Could you check a few things on this model? Use its own coordinates, in mm. A direction names the side the tool comes from. Round coordinates to 2 decimals unless told otherwise and drop trailing zeros. Loops run counter-clockwise (first coordinate to the right, second up) from the corner with the lowest first, then second, coordinate; pieces in that order, holes last. Notation, with made-up numbers: M -5.5,85 L 20.5,85 A20 ccw 20.5,103 Z; hole C 51.25,-19 d4. An arc over 180 degrees is marked long. Answer in a Markdown table with one row per item.
```python
from build123d import *

# Parameters (mm, degrees)
BASE_FLANGE1_DEPTH           = 1
SKETCH6_R                    = 6.5
CUT_EXTRUDE1_DEPTH           = 10
EDGE_FLANGE1_STRIP_W         = 10
EDGE_FLANGE1_STRIP_H         = 1
EDGE_FLANGE1_STRIP_CUT_DEPTH = 32
EDGE_FLANGE1_DEPTH           = 32
EDGE_FLANGE2_STRIP_W         = 10
EDGE_FLANGE2_STRIP_H         = 1
EDGE_FLANGE2_STRIP_CUT_DEPTH = 32
EDGE_FLANGE2_DEPTH           = 32
EDGE_FLANGE2_FLAT_DEPTH      = 1
EDGE_FLANGE3_STRIP_W         = 10
EDGE_FLANGE3_STRIP_H         = 1
EDGE_FLANGE3_STRIP_CUT_DEPTH = 8
EDGE_FLANGE3_DEPTH           = 8
EDGE_FLANGE4_STRIP_W         = 10
EDGE_FLANGE4_STRIP_H         = 1
EDGE_FLANGE4_STRIP_CUT_DEPTH = 25
EDGE_FLANGE4_DEPTH           = 25
EDGE_FLANGE4_FLAT_DEPTH      = 1
EDGE_FLANGE5_STRIP_W         = 10
EDGE_FLANGE5_STRIP_H         = 1
EDGE_FLANGE5_STRIP_CUT_DEPTH = 19
EDGE_FLANGE5_DEPTH           = 19
EDGE_FLANGE5_PROFILE_W       = 19
EDGE_FLANGE5_PROFILE_H       = 26
EDGE_FLANGE5_PROFILE_R       = 4
EDGE_FLANGE5_FLAT_DEPTH      = 1


# Sheet-metal steps are written as plain solids
with BuildPart() as part:
    # Sketch1 → Base-Flange1 (new body)
    with BuildSketch(Plane.XY):
        with BuildLine():
            Line((-47.5, 0), (47.5, 0))
            Line((47.5, 0), (47.5, -32))
            Line((47.5, -32), (31.5, -32))
            ThreePointArc((31.5, -32), (28.671572875, -33.171572875), (27.5, -36))
            Line((27.5, -36), (27.5, -44))
            Line((27.5, -44), (2.5, -44))
            Line((2.5, -44), (2.5, -30))
            ThreePointArc((2.5, -30), (1.328427125, -27.171572875), (-1.5, -26))
            Line((-1.5, -26), (-13.5, -26))
            ThreePointArc((-13.5, -26), (-16.328427125, -27.171572875), (-17.5, -30))
            Line((-17.5, -30), (-17.5, -44))
            Line((-17.5, -44), (-25.5, -44))
            Line((-25.5, -44), (-25.5, -36))
            ThreePointArc((-25.5, -36), (-26.671572875, -33.171572875), (-29.5, -32))
            Line((-29.5, -32), (-47.5, -32))
            Line((-47.5, -32), (-47.5, 0))
        make_face()
    extrude(amount=-BASE_FLANGE1_DEPTH)

    # Sketch6 → Cut-Extrude1 (cut)
    with BuildSketch(Plane.XY):
        with Locations((21, -22)):
            Circle(SKETCH6_R)
    extrude(amount=-CUT_EXTRUDE1_DEPTH, mode=Mode.SUBTRACT)

    # Edge-Flange1 strip (across the edge) → Edge-Flange1 strip cut (cut)
    with BuildSketch(Plane(origin=(47.5, 0, -1), x_dir=(-1, 0, 0), z_dir=(0, -1, 0))):
        with Locations((-1, -0.5)):
            Rectangle(EDGE_FLANGE1_STRIP_W, EDGE_FLANGE1_STRIP_H)
    edge_flange1_strip_cut = extrude(amount=EDGE_FLANGE1_STRIP_CUT_DEPTH, mode=Mode.SUBTRACT)

    # Edge-Flange1 section (across the edge) → Edge-Flange1 (add)
    with BuildSketch(Plane(origin=(47.5, 0, -1), x_dir=(-1, 0, 0), z_dir=(0, -1, 0))):
        with BuildLine():
            Line((0, 3), (0, 40))
            Line((0, 40), (1, 40))
            Line((1, 40), (1, 3))
            ThreePointArc((1, 3), (1.878679656, 0.878679656), (4, 0))
            Line((4, 0), (4, -1))
            ThreePointArc((4, -1), (1.171572875, 0.171572875), (0, 3))
        make_face()
    edge_flange1 = extrude(amount=EDGE_FLANGE1_DEPTH)

    # Edge-Flange2 strip (across the edge) → Edge-Flange2 strip cut (cut)
    with BuildSketch(Plane(origin=(47.5, -32, -41), x_dir=(0, 0, 1), z_dir=(0, 1, 0))):
        with Locations((-1, -0.5)):
            Rectangle(EDGE_FLANGE2_STRIP_W, EDGE_FLANGE2_STRIP_H)
    edge_flange2_strip_cut = extrude(amount=EDGE_FLANGE2_STRIP_CUT_DEPTH, mode=Mode.SUBTRACT)

    # Edge-Flange2 bend section (across the edge) → Edge-Flange2 (add)
    with BuildSketch(Plane(origin=(47.5, -32, -41), x_dir=(0, 0, 1), z_dir=(0, 1, 0))):
        with BuildLine():
            Line((0, 3), (1, 3))
            ThreePointArc((1, 3), (1.878679656, 0.878679656), (4, 0))
            Line((4, 0), (4, -1))
            ThreePointArc((4, -1), (1.171572875, 0.171572875), (0, 3))
        make_face()
    edge_flange2 = extrude(amount=EDGE_FLANGE2_DEPTH)

    # Edge-Flange2 profile (on flange) → Edge-Flange2 flat (add)
    with BuildSketch(Plane(origin=(47.5, 0, -41), x_dir=(0, 1, 0), z_dir=(0, 0, -1))):
        with BuildLine():
            Line((-32, 3), (0, 3))
            Line((0, 3), (0, 14))
            ThreePointArc((0, 14), (-2.050252532, 18.949747468), (-7, 21))
            Line((-7, 21), (-25, 21))
            ThreePointArc((-25, 21), (-29.949747468, 18.949747468), (-32, 14))
            Line((-32, 14), (-32, 3))
        make_face()
    edge_flange2_flat = extrude(amount=-EDGE_FLANGE2_FLAT_DEPTH)

    # Mirror1: Edge-Flange1 strip cut, Edge-Flange1, Edge-Flange2 strip cut, Edge-Flange2, Edge-Flange2 flat across plane
    add(edge_flange1_strip_cut.mirror(Plane(origin=(0, 0, 0), x_dir=(0, 0, 1), z_dir=(1, 0, 0))), mode=Mode.SUBTRACT)
    add(edge_flange1.mirror(Plane(origin=(0, 0, 0), x_dir=(0, 0, 1), z_dir=(1, 0, 0))))
    add(edge_flange2_strip_cut.mirror(Plane(origin=(0, 0, 0), x_dir=(0, 0, 1), z_dir=(1, 0, 0))), mode=Mode.SUBTRACT)
    add(edge_flange2.mirror(Plane(origin=(0, 0, 0), x_dir=(0, 0, 1), z_dir=(1, 0, 0))))
    add(edge_flange2_flat.mirror(Plane(origin=(0, 0, 0), x_dir=(0, 0, 1), z_dir=(1, 0, 0))))

    # Edge-Flange3 strip (across the edge) → Edge-Flange3 strip cut (cut)
    with BuildSketch(Plane(origin=(-17.5, -44, -1), x_dir=(0, 1, 0), z_dir=(-1, 0, 0))):
        with Locations((-1, -0.5)):
            Rectangle(EDGE_FLANGE3_STRIP_W, EDGE_FLANGE3_STRIP_H)
    extrude(amount=EDGE_FLANGE3_STRIP_CUT_DEPTH, mode=Mode.SUBTRACT)

    # Edge-Flange3 section (across the edge) → Edge-Flange3 (add)
    with BuildSketch(Plane(origin=(-17.5, -44, -1), x_dir=(0, 1, 0), z_dir=(-1, 0, 0))):
        with BuildLine():
            Line((0, 3), (0, 18))
            Line((0, 18), (1, 18))
            Line((1, 18), (1, 3))
            ThreePointArc((1, 3), (1.878679656, 0.878679656), (4, 0))
            Line((4, 0), (4, -1))
            ThreePointArc((4, -1), (1.171572875, 0.171572875), (0, 3))
        make_face()
    extrude(amount=EDGE_FLANGE3_DEPTH)

    # Edge-Flange4 strip (across the edge) → Edge-Flange4 strip cut (cut)
    with BuildSketch(Plane(origin=(27.5, -44, -1), x_dir=(0, 1, 0), z_dir=(-1, 0, 0))):
        with Locations((-1, -0.5)):
            Rectangle(EDGE_FLANGE4_STRIP_W, EDGE_FLANGE4_STRIP_H)
    extrude(amount=EDGE_FLANGE4_STRIP_CUT_DEPTH, mode=Mode.SUBTRACT)

    # Edge-Flange4 bend section (across the edge) → Edge-Flange4 (add)
    with BuildSketch(Plane(origin=(27.5, -44, -1), x_dir=(0, 1, 0), z_dir=(-1, 0, 0))):
        with BuildLine():
            Line((0, 3), (1, 3))
            ThreePointArc((1, 3), (1.878679656, 0.878679656), (4, 0))
            Line((4, 0), (4, -1))
            ThreePointArc((4, -1), (1.171572875, 0.171572875), (0, 3))
        make_face()
    extrude(amount=EDGE_FLANGE4_DEPTH)

    # Edge-Flange4 profile (on flange) → Edge-Flange4 flat (add)
    with BuildSketch(Plane(origin=(0, -44, -1), x_dir=(-1, 0, 0), z_dir=(0, -1, 0))):
        Polygon((-27.5, 3), (-2.5, 3), (-2.5, 8), (10.5, 8), (10.5, 14.535898385), (4.5, 18), (-2.5, 18), (-8.5, 18), (-8.5, 50), (-27.5, 50), align=None)
    extrude(amount=-EDGE_FLANGE4_FLAT_DEPTH)

    # Edge-Flange5 strip (across the edge) → Edge-Flange5 strip cut (cut)
    with BuildSketch(Plane(origin=(27.5, -43, -51), x_dir=(0, 0, 1), z_dir=(-1, 0, 0))):
        with Locations((-1, -0.5)):
            Rectangle(EDGE_FLANGE5_STRIP_W, EDGE_FLANGE5_STRIP_H)
    extrude(amount=EDGE_FLANGE5_STRIP_CUT_DEPTH, mode=Mode.SUBTRACT)

    # Edge-Flange5 bend section (across the edge) → Edge-Flange5 (add)
    with BuildSketch(Plane(origin=(27.5, -43, -51), x_dir=(0, 0, 1), z_dir=(-1, 0, 0))):
        with BuildLine():
            Line((0, 3), (1, 3))
            ThreePointArc((1, 3), (1.878679656, 0.878679656), (4, 0))
            Line((4, 0), (4, -1))
            ThreePointArc((4, -1), (1.171572875, 0.171572875), (0, 3))
        make_face()
    extrude(amount=EDGE_FLANGE5_DEPTH)

    # Edge-Flange5 profile (on flange) → Edge-Flange5 flat (add)
    with BuildSketch(Plane(origin=(0, -43, -51), x_dir=(-1, 0, 0), z_dir=(0, 0, -1))):
        with Locations((-18, 16)):
            Rectangle(EDGE_FLANGE5_PROFILE_W, EDGE_FLANGE5_PROFILE_H)
        with Locations((-18, 21)):
            Circle(EDGE_FLANGE5_PROFILE_R, mode=Mode.SUBTRACT)
    extrude(amount=-EDGE_FLANGE5_FLAT_DEPTH)


solid = part.part
```
1) I want a section at B-B, the plane x = 18. Please give me the cut outline in (y, z), plus the area to 3 significant figures.
Computed:
| item | result |
|---|---|
| outline | M -44,-47 A4 ccw -40,-51 L -26,-51 L -26,-50 L -40,-50 A3 cw -43,-47 L -43,-4 A3 cw -40,-1 L -27.77,-1 L -27.77,0 L -40,0 A4 ccw -44,-4 Z; M -18,-51 L -14,-51 L -14,-50 L -18,-50 Z; M -16.23,-1 L 0,-1 L 0,0 L -16.23,0 Z |
| area | 100 mm² |
2) I need wall thicknesses on line 1 (X direction, y = -19.5, z = -17); line 2 (Z direction, x = 63.5, y = -22.5); line 3 (Z direction, x = -4, y = -5). Which ranges of each line are inside material? Lowest first, please.
Computed:
| item | result |
|---|---|
| line 1 | x = -47.5 to -46.5, 46.5 to 47.5 |
| line 2 | z = -41 to -40 |
| line 3 | z = -1 to 0 |
3) If we mould it in two halves opening along Y, with no side actions, what happens to faces 4 (the face through (-66.5, -29.9, -40.5)), 5 (the face through (18.521, -18.034, -50.507)), 6 (the face through (18, -27, -51))? For each: released by +Y, released by -Y, zero draft, split by the parting line, or undercut.
Computed:
| item | result |
|---|---|
| face 4 | released by -Y |
| face 5 | undercut |
| face 6 | zero draft |
4) I want a section at D-D, the plane y = -4. Please give me the cut outline in (x, z).
Computed:
| item | result |
|---|---|
| outline | M -67.82,-41 L -50.5,-41 A4 ccw -46.5,-37 L -46.5,-4 A3 cw -43.5,-1 L 43.5,-1 A3 cw 46.5,-4 L 46.5,-37 A4 ccw 50.5,-41 L 67.82,-41 L 67.82,-40 L 50.5,-40 A3 cw 47.5,-37 L 47.5,-4 A4 ccw 43.5,0 L -43.5,0 A4 ccw -47.5,-4 L -47.5,-37 A3 cw -50.5,-40 L -67.82,-40 Z |
5) Will these pins go through, and if not, where does the flat tip stop? P1, Ø20, axis at x = 55.5, y = -17, coming from the +Z side; P2, Ø2, axis at y = -31, z = -14, coming from the +X side; P3, Ø12, axis at x = -14.5, y = -21, coming from the -Z side; P4, Ø8, axis at x = 47, z = -14, coming from the +Y side.
Computed:
| item | result |
|---|---|
| P1 | stops at z = -0.54 |
| P2 | stops at x = 47.5 |
| P3 | stops at z = -1 |
| P4 | stops at y = 0 |
6) I want a section at C-C, the plane y = -34. Please give me the cut outline in (x, z).
Computed:
| item | result |
|---|---|
| outline | M -26.04,-1 L -17.5,-1 L -17.5,0 L -26.04,0 Z; M 2.5,-1 L 28.04,-1 L 28.04,0 L 2.5,0 Z; M 8.5,-51 L 27.5,-51 L 27.5,-50 L 8.5,-50 Z |
7) I want a section at A-A, the plane y = -22. State how many separate pieces and enclosed holes the cut face has, plus the area to 3 significant figures.
Computed:
| item | result |
|---|---|
| separate pieces | 4 |
| enclosed holes | 0 |
| area | 209 mm² |
8) Which directions (+Z, -Z, +X, -X, +Y, -Y) give clear straight access to the entire face, cutting with the end or side of a thin tool? Please do faces 1 (the face through (-60, -16, -40)), 2 (the face through (47.5, -16, -20)), 3 (the face through (-21, -43, -12)).
Computed:
| item | result |
|---|---|
| face 1 | +Z, -X, +Y, -Y |
| face 2 | +Z, +X, +Y, -Y |
| face 3 | -Z, +X, -X, +Y |
